from build123d import *

# Parameters (mm, degrees)
ESQUISSE1_W             = 8
ESQUISSE1_H             = 3.6
BOSS_EXTRU_1_DEPTH      = 0.15
ESQUISSE2_W             = 7.1
ESQUISSE2_H             = 2.5
BOSS_EXTRU_2_DEPTH      = 0.85
ESQUISSE3_W             = 4.1
ESQUISSE3_H             = 0.2
BOSS_EXTRU_3_DEPTH      = 0.7
ESQUISSE4_W             = 6.6
ESQUISSE4_H             = 1.7
ENL_V_MAT_EXTRU_1_DEPTH = 0.1


with BuildPart() as part:
    # Esquisse1 → Boss.-Extru.1 (new body)
    with BuildSketch(Plane(origin=(0, 0, 0), x_dir=(1, 0, 0), z_dir=(0, 1, 0))):
        Rectangle(ESQUISSE1_W, ESQUISSE1_H)
    extrude(amount=BOSS_EXTRU_1_DEPTH)

    # Esquisse2 → Boss.-Extru.2 (add)
    with BuildSketch(Plane(origin=(0, 0.15, 0), x_dir=(1, 0, 0), z_dir=(0, 1, 0))):
        with Locations((0.05, 0.15)):
            Rectangle(ESQUISSE2_W, ESQUISSE2_H)
    extrude(amount=BOSS_EXTRU_2_DEPTH)

    # Esquisse3 → Boss.-Extru.3 (add)
    with BuildSketch(Plane.XZ):
        with Locations((1.35, 1.6)):
            Rectangle(ESQUISSE3_W, ESQUISSE3_H)
    extrude(amount=BOSS_EXTRU_3_DEPTH)

    # Esquisse4 → Enlèv. mat.-Extru.1 (cut)
    with BuildSketch(Plane(origin=(0, 1, 0), x_dir=(1, 0, 0), z_dir=(0, 1, 0))):
        with Locations((0.05, 0.15)):
            Rectangle(ESQUISSE4_W, ESQUISSE4_H)
    extrude(amount=-ENL_V_MAT_EXTRU_1_DEPTH, mode=Mode.SUBTRACT)


solid = part.part
Verification items for the finished model (mm, model axes). A direction names the side the tool comes from. Coordinates: 2 decimals unless noted, no trailing zeros. Order: outer loops, then holes, each group sorted by start corner. A loop starts at its lowest first (then second) coordinate and runs counter-clockwise, first axis right, second up.
1. Go/stop test with a flat-tipped pin: pin 1 Ø0.6 at (x, y) = (2, -0.5) entering from -Z. Record where the tip stops, or that it passes through.
Results found:
pin 1: stops at z = 1.5
2. Sectioned sample at B-B, the plane x = 1. Record the cut outline in (y, z).
Results found:
outline: (-0.7, 1.5) - (0, 1.5) - (0, -1.8) - (0.15, -1.8) - (0.15, -1.4) - (1, -1.4) - (1, -1) - (0.9, -1) - (0.9, 0.7) - (1, 0.7) - (1, 1.1) - (0.15, 1.1) - (0.15, 1.8) - (0, 1.8) - (0, 1.7) - (-0.7, 1.7) - close
3. Sectioned sample at A-A, the plane z = -1.25. Record the cut outline in (x, y), and give its area (4 significant figures).
Results found:
outline: (-4, 0) - (4, 0) - (4, 0.15) - (3.6, 0.15) - (3.6, 1) - (-3.5, 1) - (-3.5, 0.15) - (-4, 0.15) - close
area: 7.235 mm2
4. Sectioned sample at D-D, the plane z = 0.35. Record the cut outline in (x, y).
Results found:
outline: (-4, 0) - (4, 0) - (4, 0.15) - (3.6, 0.15) - (3.6, 1) - (3.35, 1) - (3.35, 0.9) - (-3.25, 0.9) - (-3.25, 1) - (-3.5, 1) - (-3.5, 0.15) - (-4, 0.15) - close
5. Sectioned sample at C-C, the plane y = -0.3. Record the cut outline in (x, z), and give its area (3 significant figures).
Results found:
outline: (-0.7, 1.5) - (3.4, 1.5) - (3.4, 1.7) - (-0.7, 1.7) - close
area: 0.820 mm2
6. Release check for a two-part mould opening along X. For faces 4 (the face through (0, 0.9, 0)), 5 (the face through (3.6, 0.6, -0.1)), 6 (the face through (0, 0, 0)), 7 (the face through (-3.5, 0.6, -0.1)) record: +X half, -X half, draft (parallel to the pull), parting line (faces both ways), or undercut.
Results found:
face 4: undercut
face 5: +X half
face 6: draft
face 7: -X half
7. Scan lines: line 1 (Y direction, x = -0.25, z = -0.1); line 2 (Y direction, x = 1, z = -1.45); line 3 (X direction, y = 0.3, z = -0.55). Record each from-to range of solid material in increasing order.
Results found:
line 1: y = 0 to 0.9
line 2: y = 0 to 0.15
line 3: x = -3.5 to 3.6
8. Set-up check for faces 1 (the face through (0, 0.6, 1.1)), 2 (the face through (0, 1, 0.9)), 3 (the face through (0, 0.6, -1.4)): record each of +Z, -Z, +X, -X, +Y, -Y from which the full face is reachable in a straight line by a thin tool's end or side.
Results found:
face 1: +Z, +X, -X, +Y
face 2: +Z, -Z, +X, -X, +Y
face 3: -Z, +X, -X, +Y
